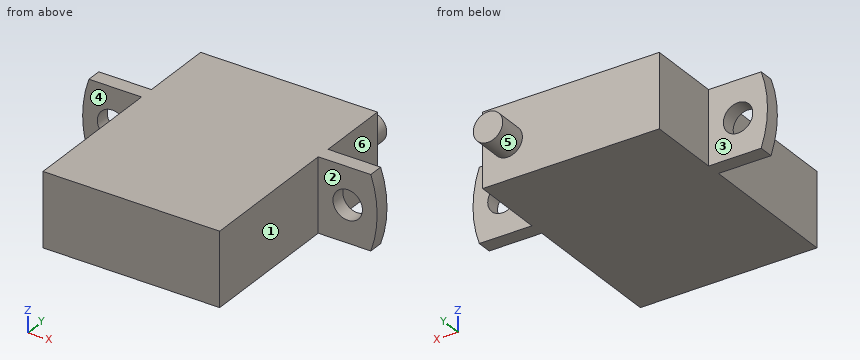
from build123d import *

# Parameters (mm, degrees)
SKETCH1_W           = 12
SKETCH1_H           = 5
BOSS_EXTRUDE1_DEPTH = 10
SKETCH2_R           = 1
SKETCH2_W           = 12
SKETCH2_H           = 5
BOSS_EXTRUDE2_DEPTH = 1
SKETCH3_W           = 12
SKETCH3_H           = 5
BOSS_EXTRUDE3_DEPTH = 5
SKETCH4_R           = 1
BOSS_EXTRUDE4_DEPTH = 2


with BuildPart() as part:
    # Sketch1 → Boss-Extrude1 (new body)
    with BuildSketch(Plane(origin=(0, 0, 0), x_dir=(1, 0, 0), z_dir=(0, 1, 0))):
        Rectangle(SKETCH1_W, SKETCH1_H)
    extrude(amount=-BOSS_EXTRUDE1_DEPTH)

    # Sketch2 → Boss-Extrude2 (add)
    with BuildSketch(Plane(origin=(0, 0, 0), x_dir=(1, 0, 0), z_dir=(0, 1, 0))):
        with BuildLine():
            Line((6, -2.5), (9.571067871, -2.5))
            ThreePointArc((9.571067871, -2.5), (10, 1e-08), (9.571067753, 2.5))
            Line((9.571067753, 2.5), (6, 2.5))
            Line((6, 2.5), (6, -2.5))
        make_face()
        with Locations((8, -5.35e-07)):
            Circle(SKETCH2_R, mode=Mode.SUBTRACT)
        Rectangle(SKETCH2_W, SKETCH2_H)
        with BuildLine():
            ThreePointArc((-9.571067871, -2.5), (-10, 1e-08), (-9.571067753, 2.5))
            Line((-9.571067753, 2.5), (-6, 2.5))
            Line((-6, 2.5), (-6, -2.5))
            Line((-6, -2.5), (-9.571067871, -2.5))
        make_face()
        with Locations((-8, -5.35e-07)):
            Circle(SKETCH2_R, mode=Mode.SUBTRACT)
    extrude(amount=BOSS_EXTRUDE2_DEPTH)

    # Sketch3 → Boss-Extrude3 (add)
    with BuildSketch(Plane(origin=(0, 1, 0), x_dir=(1, 0, 0), z_dir=(0, 1, 0))):
        Rectangle(SKETCH3_W, SKETCH3_H)
    extrude(amount=BOSS_EXTRUDE3_DEPTH)

    # Sketch4 → Boss-Extrude4 (add)
    with BuildSketch(Plane(origin=(0, 6, 0), x_dir=(1, 0, 0), z_dir=(0, 1, 0))):
        with Locations((4.297757617, 0)):
            Circle(SKETCH4_R)
    extrude(amount=BOSS_EXTRUDE4_DEPTH)


solid = part.part
Design review of the part built by this model. Coordinates are the model's own, in mm. Face numbers are marked on the shaded views. A direction names the side the tool comes from. Coordinates: 2 decimals unless noted, no trailing zeros. Write each loop counter-clockwise with the first axis right and the second up, starting at its lowest first coordinate (ties: lowest second). Pieces come first, ordered by that corner, then holes. Notation, with made-up numbers: (-37.75, 74) - (9.25, 74) arc R30 ccw to (9.25, 101) - close; hole circle Ø1 at (20.25, -37.75). An arc over 180 degrees is marked (long way). One line per item, written item: value.
1) Add section C-C (x = 4.5). State the section outline as (y, z) points.
Answer sheet:
outline: (-10, -2.5) - (6, -2.5) - (6, -0.98) - (8, -0.98) - (8, 0.98) - (6, 0.98) - (6, 2.5) - (-10, 2.5) - close
2) Add section A-A (z = 0). State the section outline as (x, y) points.
Answer sheet:
outline: (-10, 0) - (-9, 0) - (-9, 1) - (-10, 1) - close; (-7, 0) - (-6, 0) - (-6, -10) - (6, -10) - (6, 0) - (7, 0) - (7, 1) - (6, 1) - (6, 6) - (5.3, 6) - (5.3, 8) - (3.3, 8) - (3.3, 6) - (-6, 6) - (-6, 1) - (-7, 1) - close; (9, 0) - (10, 0) - (10, 1) - (9, 1) - close
3) To check wall thickness, follow probe 1 along Z at (x, y) = (-8, 0.6); probe 2 along Y at (x, z) = (9.25, 1.75); probe 3 along Y at (x, z) = (-5.75, 1.8). State the ranges of each line that lie inside material, in increasing order.
Answer sheet:
probe 1: z = -2.5 to -1, 1 to 2.5
probe 2: y = 0 to 1
probe 3: y = -10 to 6
4) Insertion check: pin 1 (2 mm diameter, centred on x = -7.5, z = 1, fed in from -Y); pin 2 (2 mm diameter, centred on x = -9, z = -0.5, fed in from +Y); pin 3 (1.6 mm diameter, centred on x = 8, z = 0, fed in from +Y); pin 4 (2.5 mm diameter, centred on y = -4, z = -1, fed in from +X). Each pin has a flat end and moves straight along its axis. Give the tip position at first contact, or say it passes through.
Answer sheet:
pin 1: stops at y = 0
pin 2: stops at y = 1
pin 3: passes through
pin 4: stops at x = 6
5) For the marked faces 4, 5 and 6, list the 3-axis set-ups (+Z, -Z, +X, -X, +Y, -Y) from which the entire face can be reached by the end or side of a thin tool; tool diameter is ignored.
Answer sheet:
face 4: +Z, -Z, -X, -Y
face 5: +Y
face 6: +Z, -Z, +X, +Y
6) Add section B-B (x = -8). State the section outline as (y, z) points, plus the area to 3 significant figures.
Answer sheet:
outline: (0, -2.5) - (1, -2.5) - (1, -1) - (0, -1) - close; (0, 1) - (1, 1) - (1, 2.5) - (0, 2.5) - close
area: 3.00 mm2
7) Mouldability with a two-part tool opening along Y and no side actions: class the marked faces 1, 2 and 3 as +Y half, -Y half, draft (parallel to the pull), parting line (faces both ways), or undercut.
Answer sheet:
face 1: draft
face 2: -Y half
face 3: +Y half
8) Add section D-D (y = 5.25). State the section outline as (x, z) points, plus the area to 3 significant figures.
Answer sheet:
outline: (-6, -2.5) - (6, -2.5) - (6, 2.5) - (-6, 2.5) - close
area: 60.0 mm2
